```python
from build123d import *

# Parameters (mm, degrees)
SKETCH_1_R           = 3
SKETCH_1_R_2         = 1.55
EXTRUDE_1_DEPTH      = 5
EXTRUDE_2_DEPTH      = 4
EXTRUDE_2_DEPTH_BACK = 3
SKETCH_2_R           = 1.3
FILLET_1_R           = 8
FILLET_2_R           = 3
CUT_EXTRUDE_1_REACH  = 62.544
SKETCH_3_R           = 3.421397557
CUT_EXTRUDE_2_DEPTH  = 1.7
FILLET_START         = 2
FILLET_3_DEPTH       = 3


with BuildPart() as part:
    # 草图1 → 凸台-拉伸1 (new body)
    with BuildSketch(Plane.XY):
        Polygon((-12.5, 0), (-18.5, 0), (-18.5, 42.034916596), (0, 60.534916596), (18.5, 42.034916596), (18.5, 0), (12.5, 0), (12.5, 35), (-12.5, 35), align=None)
        with Locations((0, 50.421397557)):
            Circle(SKETCH_1_R, mode=Mode.SUBTRACT)
        with Locations((-15.5, 5)):
            Circle(SKETCH_1_R_2, mode=Mode.SUBTRACT)
        with Locations((-15.5, 26)):
            Circle(SKETCH_1_R_2, mode=Mode.SUBTRACT)
        with Locations(Location((15.5, 5, 0), (0, 0, 180))):
            Circle(SKETCH_1_R_2, mode=Mode.SUBTRACT)
        with Locations(Location((15.5, 26, 0), (0, 0, 180))):
            Circle(SKETCH_1_R_2, mode=Mode.SUBTRACT)
    extrude(amount=EXTRUDE_1_DEPTH)

    # 草图2 → 凸台-拉伸2 (add, two sides: drawn at the far end of the back side and taken through both)
    # profile 1 of 2: a face of its own
    with BuildSketch(Plane.XY.offset(5).offset(-EXTRUDE_2_DEPTH_BACK)):
        with BuildLine():
            Line((17.5, 47), (3.906515802, 47))
            ThreePointArc((3.906515802, 47), (5.192959363, 50.421397557), (3.906515802, 53.842795113))
            Line((3.906515802, 53.842795113), (17.5, 53.842795113))
            Line((17.5, 53.842795113), (17.5, 47))
        make_face()
        with Locations(Location((12.5, 50.421397557, 0), (0, 0, 180))):
            Circle(SKETCH_2_R, mode=Mode.SUBTRACT)
    # profile 2 of 2: a face of its own
    with BuildSketch(Plane.XY.offset(5).offset(-EXTRUDE_2_DEPTH_BACK)):
        with BuildLine():
            Line((-17.5, 47), (-17.5, 53.842795113))
            Line((-17.5, 53.842795113), (-3.906515802, 53.842795113))
            ThreePointArc((-3.906515802, 53.842795113), (-5.192959363, 50.421397557), (-3.906515802, 47))
            Line((-3.906515802, 47), (-17.5, 47))
        make_face()
        with Locations((-12.5, 50.421397557)):
            Circle(SKETCH_2_R, mode=Mode.SUBTRACT)
    extrude(amount=EXTRUDE_2_DEPTH + EXTRUDE_2_DEPTH_BACK)

    # 圆角1
    fillet_1_edges = [part.edges().sort_by_distance(p)[0] for p in [
        (-18.5, 42.034916596, 2.5),
        (0, 60.534916596, 2.5),
        (18.5, 42.034916596, 2.5),
    ]]
    fillet(fillet_1_edges, radius=FILLET_1_R)

    # 圆角2
    fillet_2_edges = [part.edges().sort_by_distance(p)[0] for p in [
        (-6.692121483, 53.842795113, 3.5),
        (-17.5, 47, 5.5),
        (-5.192959363, 50.421397557, 9),
        (-17.5, 53.842795113, 5.5),
        (6.692121483, 53.842795113, 3.5),
        (17.5, 53.842795113, 5.5),
        (5.192959363, 50.421397557, 9),
        (17.5, 47, 5.5),
    ]]
    fillet(fillet_2_edges, radius=FILLET_2_R)

    # 草图3 → 切除-拉伸1 (cut, up to next)
    with BuildSketch(Plane(origin=(0, 0, 2), x_dir=(-1, 0, 0), z_dir=(0, 0, -1)), mode=Mode.PRIVATE) as cut_extrude_1_sk1:
        with Locations((-12.5, 50.421397557)):
            Circle(SKETCH_3_R)
    cut_extrude_1_tool1 = extrude(cut_extrude_1_sk1.sketch, amount=CUT_EXTRUDE_1_REACH, mode=Mode.PRIVATE) & part.part
    # 草图3 → 切除-拉伸1 (cut, up to next)
    with BuildSketch(Plane(origin=(0, 0, 2), x_dir=(-1, 0, 0), z_dir=(0, 0, -1)), mode=Mode.PRIVATE) as cut_extrude_1_sk2:
        with Locations((12.5, 50.421397557)):
            Circle(SKETCH_3_R)
    cut_extrude_1_tool2 = extrude(cut_extrude_1_sk2.sketch, amount=CUT_EXTRUDE_1_REACH, mode=Mode.PRIVATE) & part.part
    add(cut_extrude_1_tool1.solids().sort_by_distance((12.5, 50.421398, 2))[0], mode=Mode.SUBTRACT)
    add(cut_extrude_1_tool2.solids().sort_by_distance((-12.5, 50.421398, 2))[0], mode=Mode.SUBTRACT)

    # 草图4 → 切除-拉伸2 (cut)
    with BuildSketch(Plane.XY.offset(9)):
        Polygon((0, 46.899022366), (43.079074711, 50.891584803), (0, 53.943772747), (-43.079074711, 50.891584803), align=None)
    extrude(amount=-CUT_EXTRUDE_2_DEPTH, mode=Mode.SUBTRACT)

    # 圆角3: read off the stored shape, not the designer's step
    # 圆角3 outline → 圆角3 (add)
    with BuildSketch(Plane.XY.offset(FILLET_START)):
        with BuildLine():
            ThreePointArc((17.623806552, 42.361452624), (16.757691875, 45.600251323), (17.294803574, 48.909553768))
            ThreePointArc((17.294803574, 48.909553768), (16.192433353, 47.52297167), (14.5, 47))
            Line((14.5, 47), (13.534916596, 47))
            Line((13.534916596, 47), (16.156854249, 44.378062347))
            ThreePointArc((16.156854249, 44.378062347), (16.969389563, 43.42726788), (17.623806552, 42.361452624))
        make_face()
        with BuildLine():
            ThreePointArc((-14.5, 47), (-16.192433353, 47.52297167), (-17.294803574, 48.909553768))
            ThreePointArc((-17.294803574, 48.909553768), (-16.757691875, 45.600251323), (-17.623806552, 42.361452624))
            ThreePointArc((-17.623806552, 42.361452624), (-16.969389563, 43.42726788), (-16.156854249, 44.378062347))
            Line((-16.156854249, 44.378062347), (-13.534916596, 47))
            Line((-13.534916596, 47), (-14.5, 47))
        make_face()
    extrude(amount=FILLET_3_DEPTH)


solid = part.part
```
Geometry check sheet. Reference: the model listing, model coordinates, mm. A direction names the side the tool comes from. Give positions to 0.01 mm unless a question says otherwise; leave off trailing zeros. Loops run counter-clockwise (first coordinate to the right, second up) from the corner with the lowest first, then second, coordinate; pieces in that order, holes last. Notation, with made-up numbers: M 48,69.5 L 78,69.5 A13 ccw 78,76.5 Z; hole C 70,55 d8. An arc over 180 degrees is marked long. Answer as CSV lines item,"result".
Item 1: Cross-section at C-C on z = 3.25. Count the separate pieces of the cut face and the enclosed holes in it, and give its area (3 significant figures).
Values:
separate pieces,"1"
enclosed holes,"7"
area,"1,040 mm²"
Item 2: Release check for a two-part mould opening along Y. For faces 5 (the cylindrical face through (-10.045, 48.038, 1.014)), 6 (the flat face through (18.5, 20, 2)), 7 (the cylindrical face through (-6.77, 54.08, 3.48)), 8 (the flat face through (0, 35, 2)) record: pulls with the +Y half, pulls with the -Y half, needs draft (parallel to the pull), parting line crosses it, or undercut.
Values:
face 5,"undercut"
face 6,"needs draft"
face 7,"pulls with the +Y half"
face 8,"pulls with the -Y half"
Item 3: Cross-section at A-A on x = 0. Record the cut outline in (y, z), and give its area (3 significant figures).
Values:
outline,"M 35,0 L 47.42,0 L 47.42,5 L 35,5 Z; M 53.42,0 L 57.22,0 L 57.22,5 L 53.42,5 Z"
area,"81.1 mm²"
Item 4: Cross-section at B-B on y = 5. Record the cut outline in (x, z).
Values:
outline,"M -18.5,0 L -17.05,0 L -17.05,5 L -18.5,5 Z; M -13.95,0 L -12.5,0 L -12.5,5 L -13.95,5 Z; M 12.5,0 L 13.95,0 L 13.95,5 L 12.5,5 Z; M 17.05,0 L 18.5,0 L 18.5,5 L 17.05,5 Z"
Item 5: Cross-section at D-D on x = -15.5. Record the cut outline in (y, z), and give its area (3 significant figures).
Values:
outline,"M 0,0 L 3.45,0 L 3.45,5 L 0,5 Z; M 6.55,0 L 24.45,0 L 24.45,5 L 6.55,5 Z; M 27.55,0 L 45.03,0 L 45.03,2 L 53.67,2 L 53.67,9 L 52.85,9 L 52.85,7.3 L 48.34,7.3 L 48.34,9 L 47.17,9 L 47.17,5 L 27.55,5 Z"
area,"238 mm²"
Item 6: Access from +Z, -Z, +X, -X, +Y, -Y to the whole of each face (thin tool, end or side, straight path). Record for faces 1 (the flat face through (-10, 53.843, 5)), 2 (the cylindrical face through (16.6, 47.86, 6.33)), 3 (the flat face through (11, 51, 7.3)), 4 (the flat face through (9, 47, 7)).
Values:
face 1,"+Z, -X, +Y"
face 2,"+Z, +X"
face 3,"+Z"
face 4,"+Z, +X, -X, -Y"
Item 7: Depth check by flat-ended pin: P1, Ø1.9, axis at x = -8.5, y = 51.5, coming from the +Z side; P2, Ø3, axis at x = 7.5, z = 5, coming from the +Y side; P3, Ø3, axis at x = -11.5, z = 7.5, coming from the -Y side; P4, Ø13, axis at x = 13.5, y = 48, coming from the -Z side. Enter the tip coordinate at first touch or a pass-through.
Values:
P1,"stops at z = 7.3"
P2,"stops at y = 54.55"
P3,"stops at y = 47"
P4,"stops at z = 0"
Item 8: Material ranges on line 1 (Y direction, x = 0, z = 3.25); line 2 (Y direction, x = -15.5, z = 2.9); line 3 (X direction, y = 19.5, z = 4.5), recorded low to high.
Values:
line 1,"y = 35 to 47.42, 53.42 to 57.22"
line 2,"y = 0 to 3.45, 6.55 to 24.45, 27.55 to 53.67"
line 3,"x = -18.5 to -12.5, 12.5 to 18.5"
